Source: CAD feature listing. Evaluate the final solid. Frame: model axes, mm. Face numbers are marked on the shaded views. A direction names the side the tool comes from. Give positions to 0.01 mm unless a question says otherwise; leave off trailing zeros. Write each loop counter-clockwise with the first axis right and the second up, starting at its lowest first coordinate (ties: lowest second). Pieces come first, ordered by that corner, then holes. Notation, with made-up numbers: (-14.5, 56.25) - (35.5, 56.25) arc R7 cw to (35.5, 68.25) - close; hole circle Ø10 at (-28, 83.5). An arc over 180 degrees is marked (long way). One line per question, with ' | ' between items. Start each with the question number.
(1) Ray query, line 1 (X direction, y = 6.25, z = 11.75); line 2 (X direction, y = 19.75, z = 15.25). Return the intervals inside material, ascending. Write a range as [from, to].
(2) Section D-D, the plane y = 14.25. Return loops of the section in (x, z), plus the area to 3 significant figures.
(3) Access query for the marked faces 1, 2 and 3. Directions: +Z, -Z, +X, -X, +Y, -Y. A direction counts if a zero-diameter tool reaches every point of the face in a straight line with its end or side. Return the directions, or none.
(4) Pin query (flat end, axial travel): pin 1 (2 mm diameter, centred on y = 19, z = 15, fed in from +X); pin 2 (7.5 mm diameter, centred on x = 10.5, z = 13, fed in from +Y); pin 3 (1.5 mm diameter, centred on x = 4.5, z = 2.5, fed in from +Y). Return the tip coordinate at first contact, or that it passes through.
(5) Section B-B, the plane z = 6. Return loops of the section in (x, y).
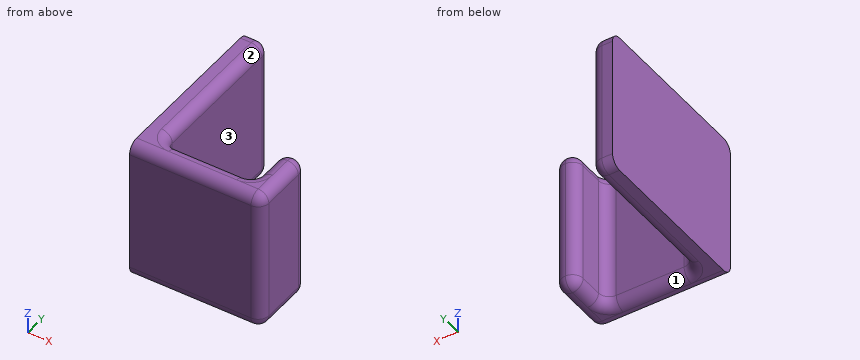
```python
from build123d import *

# Parameters (mm, degrees)
F1_DEPTH = 20
F2_R     = 1.49999


# Not quite as in the source:
# - a fillet or chamfer is up to 0.001 mm smaller than in the source, because OpenCascade refuses the exact size


with BuildPart() as f1:
    # F0 (on Top) → F1 (new body)
    with BuildSketch(Plane.XY):
        with BuildLine():
            Line((1.5, 25), (0, 25))
            Line((0, 25), (0, 0))
            Line((0, 0), (17, 0))
            ThreePointArc((17, 0), (18.0606601718, 0.4393398282), (18.5, 1.5))
            Line((18.5, 1.5), (18.5, 7.75))
            ThreePointArc((18.5, 7.75), (18.0606601718, 8.8106601718), (17, 9.25))
            ThreePointArc((17, 9.25), (15.9393398282, 8.8106601718), (15.5, 7.75))
            Line((15.5, 7.75), (15.5, 4.5))
            ThreePointArc((15.5, 4.5), (15.0606601718, 3.4393398282), (14, 3))
            Line((14, 3), (4.5, 3))
            ThreePointArc((4.5, 3), (3.4393398282, 3.4393398282), (3, 4.5))
            Line((3, 4.5), (3, 23.5))
            ThreePointArc((3, 23.5), (2.5606601718, 24.5606601718), (1.5, 25))
        make_face()
    extrude(amount=F1_DEPTH)

    # F2 (radius 1.5 in the source; OpenCascade refuses exactly that, so slightly less here)
    f2_edges = [f1.edges().sort_by_distance(p)[0] for p in [
        (3, 14, 20),
        (9.25, 3, 0),
    ]]
    fillet(f2_edges, radius=F2_R)


solid = f1.part
```
Check sheet entries:
1) line 1: [0, 3], [15.5, 18.5] | line 2: [0, 3]
2) outline: (0, 0) - (1.5, 0) arc R1.5 ccw to (3, 1.5) - (3, 18.5) arc R1.5 ccw to (1.5, 20) - (0, 20) - close | area: 59.0 mm²
3) face 1: -Z, +Y | face 2: +Z, +Y | face 3: +Z, -Z, +Y
4) pin 1: x = 3 | pin 2: y = 3.02 | pin 3: y = 3.2
5) outline: (0, 0) - (17, 0) arc R1.5 ccw to (18.5, 1.5) - (18.5, 7.75) arc R1.5 ccw to (15.5, 7.75) - (15.5, 4.5) arc R1.5 cw to (14, 3) - (4.5, 3) arc R1.5 cw to (3, 4.5) - (3, 23.5) arc R1.5 ccw to (1.5, 25) - (0, 25) - close
